Part model, mm, in its own coordinate system. Face numbers are marked on the shaded views. Give positions to 0.01 mm unless a question says otherwise; leave off trailing zeros. Order: outer loops, then holes, each group sorted by start corner. A loop starts at its lowest first (then second) coordinate and runs counter-clockwise, first axis right, second up. Notation, with made-up numbers: M 75,-3.5 L 104,-3.5 A17 ccw 104,23.5 Z; hole C 78,-25.75 d9. An arc over 180 degrees is marked long. Answer as a JSON object with one key per item and string values.
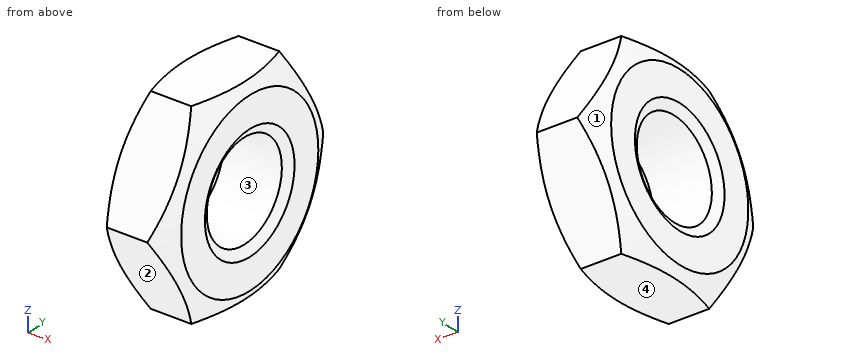
Autodesk Inventor part; units mm, degrees
ref_plane "Work Plane1" through (-20.7291, 0, 0) normal (0, -0.866, -0.5) x (1, 0, 0)
ref_plane "YZ Plane" through (0, 0, 0) normal (1, 0, 0) x (0, 1, 0)
ref_plane "XZ Plane" through (0, 0, 0) normal (0, 1, 0) x (-1, 0, 0)
sketch "Эскиз1" plane through (0, 0, 0) normal (1, 0, 0) x (0, 1, 0)
  line L0 (-9.815, 0) -> (-4.9075, 8.5)
  line L1 (-4.9075, 8.5) -> (4.9075, 8.5)
  line L2 (4.9075, 8.5) -> (9.815, 0)
  line L3 (9.815, 0) -> (4.9075, -8.5)
  line L4 (4.9075, -8.5) -> (-4.9075, -8.5)
  line L5 (-4.9075, -8.5) -> (-9.815, 0)
  point P0 (0, 0)
  point P1 (0, 0)
  dimension "d0" = 19.6299
extrude "Базовый элемент" add sketch "Эскиз1" along normal blind 6
sketch "Эскиз2" plane through (0, 0, 0) normal (0, 0, 1) x (1, 0, 0)
  line L0 (0, 4.9075) -> (0, 9.815)
  line L1 (0, 9.815) -> (6, 9.815)
  line L2 (6, 4.9075) -> (6, 9.815)
  line L3 (-1.2, 0) -> (7.2, 0)
  line L4 (1.2499, 9.815) -> (0, 7.65)
  line L5 (4.7501, 9.815) -> (6, 7.65)
  dimension "d3" = 30
  dimension "d4" = 30
  dimension "d5" = 15.3
  dimension "d6" = 15.3
revolve "Фаска1" cut sketch "Эскиз2" angle 360 about axis through (-10, 0, 0) along (1, 0, 0)
sketch "Эскиз3" plane through (6, 0, 0) normal (1, 0, 0) x (0, 0, -1)
  arc A0 (-0.625, -1.0825) -> (0.625, -1.0825) centre (0, 0) ccw
hole "Резьба" at (6, 0, 0) direction (-1, 0, 0) diameter 8.376 end through all
chamfer "Фаска2" distance 0.8119 angle 30 1 edges at (6, 0, 4.188) measured on face at (6, 6.4117, -0.7785)
chamfer "Фаска3" distance 0.8119 angle 30 1 edges at (0, 0, 4.188) measured on face at (0, 6.4117, -0.7785)
ref_plane "Work Plane1" through (-20.7291, 0, 0) normal (0, -0.866, -0.5) x (1, 0, 0)
equation "\"d0\" = 1.1547 * SW"
equation "\"d1\" = KOH"
equation "\"d3\" = ANG1"
equation "\"d4\" = ANG2"
equation "\"d5\" = SW0"
equation "\"d6\" = SW01"
equation "\"d8\" = -0.5 * GD1 + 0.5 * NND"
equation "\"d40\" = -0.5 * GD1 + 0.5 * NND"
equation "\"d10\" = -0.5 * GD1 + 0.5 * NND"
equation "\"d41\" = -0.5 * GD1 + 0.5 * NND"
equation "\"ANG1\" = 30deg"
equation "\"ANG2\" = 30deg"
equation "\"KOH\" = 6"
equation "\"SW\" = 17"
equation "\"SW0\" = 15.3"
equation "\"SW01\" = 15.3"
equation "\"GUL\" = 0.541266 * PTC"
equation "\"LADI\" = 16.15"
equation "\"TOA\" = 30deg"
equation "\"FAWI\" = 30deg"
equation "\"PTC\" = 1.5"
equation "\"E0\" = 1.155 * SW"
equation "\"GAL\" = 0.541266 * PTC"
properties part number "Гайка M10-6H ГОСТ 5916-70" material "Сталь, мягкая"
1. Cut at C-C on x = 5.1. Give the cut face in (y, z), plus the area to 3 significant figures.
Worked answers:
{"outline": "M -9.13,-1.18 L -5.59,-7.32 A9.21 ccw -3.54,-8.5 L 3.54,-8.5 A9.21 ccw 5.59,-7.32 L 9.13,-1.18 A9.21 ccw 9.13,1.18 L 5.59,7.32 A9.21 ccw 3.54,8.5 L -3.54,8.5 A9.21 ccw -5.59,7.32 L -9.13,1.18 A9.21 ccw Z; hole C 0,0 d8.38", "area": "191 mm^2"}
2. Probe line 1 along Z through (x, y) = (2.8, 0); line 2 along Z through (x, y) = (3.6, 2.75); line 3 along Y through (x, z) = (3, -1). List the from-to ranges inside material, lowest first.
Worked answers:
{"line 1": "z = -8.5 to -4.19, 4.19 to 8.5", "line 2": "z = -8.5 to -3.16, 3.16 to 8.5", "line 3": "y = -9.24 to -4.07, 4.07 to 9.24"}
3. Pin check, flat tips, straight feed: P1, Ø3, axis at x = 1.5, z = -2.5, coming from the +Y side; P2, Ø1, axis at y = 1.5, z = 1, coming from the +X side. Stop position of each tip, or through.
Worked answers:
{"P1": "stops at y = 9.24", "P2": "passes through"}
4. Two-plate mould, pull along Y, no slides. Class the marked faces 1, 2, 3 and 4: +Y half, -Y half, draft (parallel to the pull), parting line (faces both ways), or undercut.
Worked answers:
{"face 1": "parting line", "face 2": "-Y half", "face 3": "undercut", "face 4": "draft"}
5. Cut at A-A on y = 0. Give the cut face in (x, z).
Worked answers:
{"outline": "M 0,-7.65 L 0.49,-8.5 L 5.51,-8.5 L 6,-7.65 L 6,-5 L 5.53,-4.19 L 0.47,-4.19 L 0,-5 Z; M 0,5 L 0.47,4.19 L 5.53,4.19 L 6,5 L 6,7.65 L 5.51,8.5 L 0.49,8.5 L 0,7.65 Z"}
6. Cut at B-B on x = 3.35. Give the cut face in (y, z) (1 decimal).
Worked answers:
{"outline": "M -9.8,0 L -4.9,-8.5 L 4.9,-8.5 L 9.8,0 L 4.9,8.5 L -4.9,8.5 Z; hole C 0,0 d8.4"}
